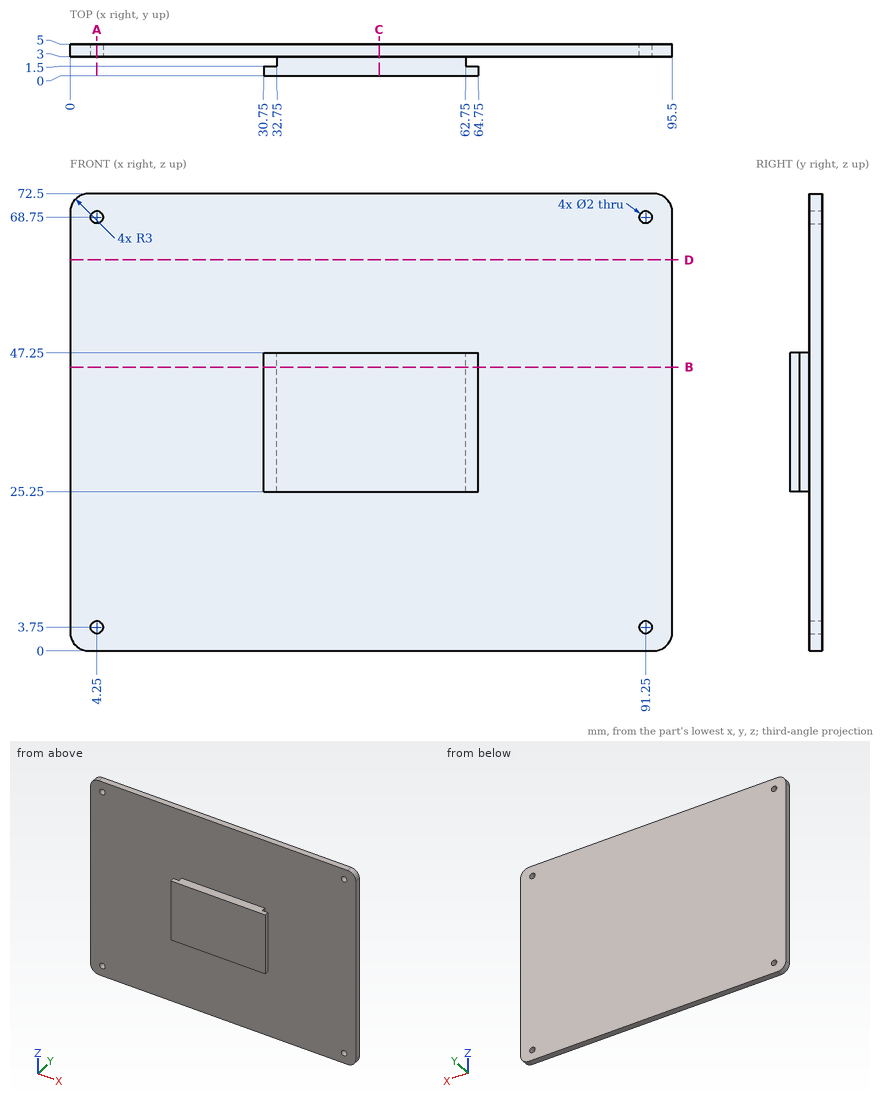
Input: dimensioned drawing with shaded views. Units: mm. Origin: part minimum x, y, z. Round coordinates to 2 decimals unless told otherwise and drop trailing zeros. Loops run counter-clockwise (first coordinate to the right, second up) from the corner with the lowest first, then second, coordinate; pieces in that order, holes last. Notation, with made-up numbers: (50, -19) -> (90, -19) arc R6 ccw to (90, -12) -> close; hole circle Ø3 at (26.25, 51). An arc over 180 degrees is marked (long way). Use one line per item in the form item = value. Start each with the question number.
1) Section C-C on x = 49. Output: boundary loops of the cut face in (y, z).
2) Line query: L1, parallel to Z at x = 91.25, y = 4.3; L2, parallel to X at y = 3.45, z = 3.75; L3, parallel to Y at x = 37, z = 21. Output: solid intervals per line, ascending.
3) Section A-A on x = 4.25. Output: boundary loops of the cut face in (y, z).
4) Section B-B on z = 45. Output: boundary loops of the cut face in (x, y), then the cut area to 3 significant figures.
5) Section D-D on z = 62. Output: boundary loops of the cut face in (x, y), then the cut area to 3 significant figures.
6) First-contact query: P1, Ø2.5, axis at x = 4.25, z = 68.75, coming from the -Y side; P2, Ø1.8, axis at x = 4.25, z = 3.75, coming from the -Y side; P3, Ø0.8, axis at y = 2, z = 33, coming from the +X side; P4, Ø0.9, axis at x = 54.5, y = 1.5, coming from the -Z side. Flat tips, straight axial feed; report the tip coordinate or a pass-through.
Response:
q1.outline = (0, 25.25) -> (3, 25.25) -> (3, 0) -> (5, 0) -> (5, 72.5) -> (3, 72.5) -> (3, 47.25) -> (0, 47.25) -> close
q2.L1 = 0 to 2.75, 4.75 to 67.75, 69.75 to 72.5
q2.L2 = 0 to 3.25, 5.25 to 90.25, 92.25 to 95.5
q2.L3 = 3 to 5
q3.outline = (3, 0) -> (5, 0) -> (5, 2.75) -> (3, 2.75) -> close; (3, 4.75) -> (5, 4.75) -> (5, 67.75) -> (3, 67.75) -> close; (3, 69.75) -> (5, 69.75) -> (5, 72.5) -> (3, 72.5) -> close
q4.outline = (0, 3) -> (32.75, 3) -> (32.75, 1.5) -> (30.75, 1.5) -> (30.75, 0) -> (64.75, 0) -> (64.75, 1.5) -> (62.75, 1.5) -> (62.75, 3) -> (95.5, 3) -> (95.5, 5) -> (0, 5) -> close
q4.area = 287 mm^2
q5.outline = (0, 3) -> (95.5, 3) -> (95.5, 5) -> (0, 5) -> close
q5.area = 191 mm^2
q6.P1 = 3
q6.P2 = through
q6.P3 = 62.75
q6.P4 = 25.25
